Geometry: final body of the model. Coordinates: model frame, mm. A direction names the side the tool comes from. Give positions to 0.01 mm unless a question says otherwise; leave off trailing zeros. Write each loop counter-clockwise with the first axis right and the second up, starting at its lowest first coordinate (ties: lowest second). Pieces come first, ordered by that corner, then holes. Notation, with made-up numbers: M -2,55 L 15,55 A23 cw 15,69 Z; hole C 24,-14 d7. An arc over 180 degrees is marked long. Use one line per item in the form item = value. Start each with the question number.
Item 1: Material intervals for line 1 along Y through (x, z) = (14, 0.35); line 2 along Y through (x, z) = (-44, 0.4); line 3 along X through (y, z) = (-2.5, 1.95), sorted ascending. Write a range as from..to.
Item 2: Access query for faces 1 (the flat face through (-5, 18.795, 1)), 2 (the flat face through (-6, -20, 0)). Directions: +Z, -Z, +X, -X, +Y, -Y. A direction counts if a zero-diameter tool reaches every point of the face in a straight line with its end or side. Return the directions, or none.
Item 3: Section query C-C on z = 1.5. Return loops of the section in (x, y), then the cut area to 3 significant figures.
Item 4: Pull-direction query (X, two-part tool) for faces 3 (the cylindrical face through (-52.15, -19.7, 1.01)), 4 (the cylindrical face through (31.9, 1.07, 0.99)), 5 (the flat face through (15.009, 2, 1)), 6 (the cylindrical face through (42, 23.46, 1.01)); classes: released by +X, released by -X, zero draft, split by the parting line, or undercut.
Item 5: Section query B-B on y = 13. Return loops of the section in (x, z), then the cut area to 3 significant figures.
Item 6: Section query A-A on x = -44. Return loops of the section in (y, z), then the cut area to 3 significant figures.
from build123d import *

# Parameters (mm, degrees)
SKETCH1_W           = 100.01257602
SKETCH1_H           = 49.015555291
SKETCH1_R           = 2.1
SKETCH1_W_2         = 39.998541852
SKETCH1_H_2         = 34.001078585
BOSS_EXTRUDE1_DEPTH = 2
FILLET1_R           = 10


with BuildPart() as part:
    # Sketch1 → Boss-Extrude1 (new body)
    with BuildSketch(Plane.XY):
        with Locations((-5, 1.804116785)):
            Rectangle(SKETCH1_W, SKETCH1_H)
        with Locations((-44, 0.98172734)):
            Circle(SKETCH1_R, mode=Mode.SUBTRACT)
        with Locations((34, 0.98172734)):
            Circle(SKETCH1_R, mode=Mode.SUBTRACT)
        with Locations((-4.990588882, 1.794943283)):
            Rectangle(SKETCH1_W_2, SKETCH1_H_2, mode=Mode.SUBTRACT)
    extrude(amount=BOSS_EXTRUDE1_DEPTH)

    # Fillet1
    fillet1_edges = [part.edges().sort_by_distance(p)[0] for p in [
        (-55.00628801, 26.311894431, 1),
        (45.00628801, 26.311894431, 1),
        (45.00628801, -22.70366086, 1),
        (-55.00628801, -22.70366086, 1),
    ]]
    fillet(fillet1_edges, radius=FILLET1_R)


solid = part.part
Answer sheet:
q1.line_1 = -22.7..-15.21, 18.8..26.31
q1.line_2 = -22.7..-1.12, 3.08..26.31
q1.line_3 = -55.01..-24.99, 15.01..45.01
q2.face_1 = +Z, -Z
q2.face_2 = -Z, +X, -X, +Y, -Y
q3.outline = M -55.01,-12.7 A10 ccw -45.01,-22.7 L 35.01,-22.7 A10 ccw 45.01,-12.7 L 45.01,16.31 A10 ccw 35.01,26.31 L -45.01,26.31 A10 ccw -55.01,16.31 Z; hole C -44,0.98 d4.2; hole M -24.99,-15.21 L 15.01,-15.21 L 15.01,18.8 L -24.99,18.8 Z; hole C 34,0.98 d4.2
q3.area = 3,430 mm2
q4.face_3 = released by -X
q4.face_4 = undercut
q4.face_5 = undercut
q4.face_6 = released by +X
q5.outline = M -55.01,0 L -24.99,0 L -24.99,2 L -55.01,2 Z; M 15.01,0 L 45.01,0 L 45.01,2 L 15.01,2 Z
q5.area = 120 mm2
q6.outline = M -22.7,0 L -1.12,0 L -1.12,2 L -22.7,2 Z; M 3.08,0 L 26.31,0 L 26.31,2 L 3.08,2 Z
q6.area = 89.6 mm2
